The listing builds one solid part. Answer for the finished solid, in the listing's coordinates (mm). Face numbers are marked on the shaded views. A direction names the side the tool comes from. Coordinates: 2 decimals unless noted, no trailing zeros. Order: outer loops, then holes, each group sorted by start corner. A loop starts at its lowest first (then second) coordinate and runs counter-clockwise, first axis right, second up.
```python
from build123d import *

# Parameters (mm, degrees)
SKETCH_W        = 64
SKETCH_H        = 100
PAD_DEPTH       = 19
SKETCH001_W     = 50
SKETCH001_H     = 12.746663
POCKET_DEPTH    = 100.001
SKETCH002_W     = 64
SKETCH002_H     = 38
PAD001_DEPTH    = 25
POCKET001_DEPTH = 13
SKETCH004_R     = 3
SKETCH004_R_2   = 5
POCKET002_DEPTH = 20
SKETCH005_R     = 5
POCKET003_DEPTH = 24.001
POCKET004_DEPTH = 19.001


with BuildPart() as part:
    # Sketch → Pad (new body)
    with BuildSketch(Plane.XY):
        Rectangle(SKETCH_W, SKETCH_H)
    extrude(amount=PAD_DEPTH)

    # Sketch001 → Pocket (cut, through all)
    with BuildSketch(Plane.XZ.offset(50)):
        with Locations((0, -0.373331)):
            Rectangle(SKETCH001_W, SKETCH001_H)
    extrude(amount=-POCKET_DEPTH, mode=Mode.SUBTRACT)

    # Sketch002 → Pad001 (new body)
    with BuildSketch(Plane.XY.offset(19)):
        with Locations((0, 31)):
            Rectangle(SKETCH002_W, SKETCH002_H)
    extrude(amount=PAD001_DEPTH)

    # Sketch003 → Pocket001 (cut)
    with BuildSketch(Plane.XY.offset(44)):
        Polygon((-12, 50), (-19, 12), (19, 12), (12, 50), align=None)
    extrude(amount=-POCKET001_DEPTH, mode=Mode.SUBTRACT)

    # Sketch004 → Pocket002 (cut)
    with BuildSketch(Plane.XY.offset(44)):
        with Locations((-22, 37)):
            Circle(SKETCH004_R)
        with Locations((22, 37)):
            Circle(SKETCH004_R)
        with Locations((0, 31)):
            Circle(SKETCH004_R_2)
    extrude(amount=-POCKET002_DEPTH, mode=Mode.SUBTRACT)

    # Sketch005 → Pocket003 (cut, through all)
    with BuildSketch(Plane.XY.offset(24)):
        with Locations((0, 31)):
            Circle(SKETCH005_R)
    extrude(amount=-POCKET003_DEPTH, mode=Mode.SUBTRACT)

    # Sketch006 → Pocket004 (cut, through all)
    with BuildSketch(Plane.XY.offset(19)):
        with BuildLine():
            ThreePointArc((9, -10), (0, -1), (-9, -10))
            Line((-9, -10), (-9, -30))
            ThreePointArc((-9, -30), (0, -39), (9, -30))
            Line((9, -10), (9, -30))
        make_face()
    extrude(amount=-POCKET004_DEPTH, mode=Mode.SUBTRACT)


solid = part.part
```
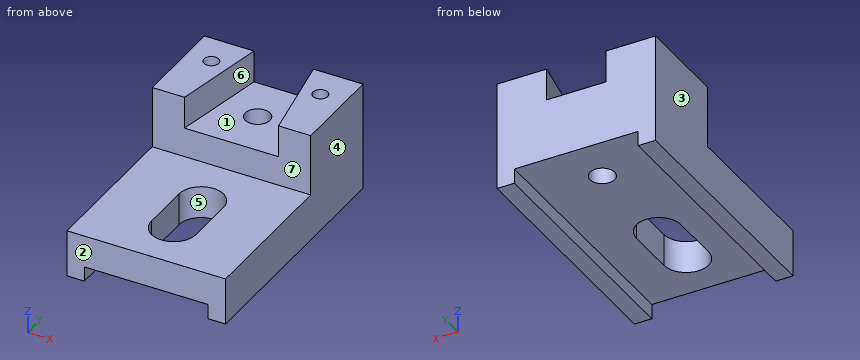
(1) The mould has two halves that part along X. Classify the marked faces 1, 2, 3 and 4: released by +X, released by -X, zero draft, split by the parting line, or undercut.
(2) Consider line 1 (Y direction, x = 0, z = 16); line 2 (Y direction, x = -22, z = 36); line 3 (X direction, y = -34.5, z = 3.5). Determine where each line is inside the solid, lowest interval first.
(3) Find section D-D (z = 13). Write down the section's boundary in (x, y), and give its area (3 significant figures).
(4) For the marked faces 5, 6 and 7, determine the directions among +Z, -Z, +X, -X, +Y, -Y from which every point of the face is accessible in a straight line to the end or side of a thin tool.
(5) Find section C-C (y = 31). Write down the section's boundary in (x, z).
(6) Each of these flat-tipped pins is pushed along its axis until it touches: pin 1 Ø8 at (x, y) = (-7.5, 19) entering from +Z; pin 2 Ø18.5 at (x, y) = (-6.5, -8.5) entering from +Z; pin 3 Ø7.5 at (x, z) = (-2.5, 31.5) entering from -Y. Where does it stop, or does it pass through?
(7) Find section B-B (x = 0). Write down the section's boundary in (y, z), and give its area (3 significant figures).
(8) Find section A-A (z = 32.5). Write down the section's boundary in (x, y).
Findings below:
1. face 1: undercut
1. face 2: zero draft
1. face 3: released by -X
1. face 4: released by +X
2. line 1: y = -50 to -39, -1 to 26, 36 to 50
2. line 2: y = 12 to 34, 40 to 50
2. line 3: x = -32 to -25, 25 to 32
3. outline: (-32, -50) - (32, -50) - (32, 50) - (-32, 50) - close; hole (-9, -30) arc R9 ccw to (9, -30) - (9, -10) arc R9 ccw to (-9, -10) - close; hole circle Ø10 at (0, 31)
3. area: 5,710 mm2
4. face 5: +Z, -Z
4. face 6: +Z, -Y
4. face 7: +Z, +X, -X, -Y
5. outline: (-32, 0) - (-25, 0) - (-25, 6) - (-5, 6) - (-5, 31) - (-15.5, 31) - (-15.5, 44) - (-32, 44) - close; (5, 6) - (25, 6) - (25, 0) - (32, 0) - (32, 44) - (15.5, 44) - (15.5, 31) - (5, 31) - close
6. pin 1: stops at z = 31
6. pin 2: stops at z = 19
6. pin 3: stops at y = 12
7. outline: (-50, 6) - (-39, 6) - (-39, 19) - (-50, 19) - close; (-1, 6) - (26, 6) - (26, 31) - (12, 31) - (12, 19) - (-1, 19) - close; (36, 6) - (50, 6) - (50, 31) - (36, 31) - close
7. area: 1,010 mm2
8. outline: (-32, 12) - (-19, 12) - (-12, 50) - (-32, 50) - close; (12, 50) - (19, 12) - (32, 12) - (32, 50) - close; hole circle Ø6 at (-22, 37); hole circle Ø6 at (22, 37)
